For this review, take the finished solid that the model builds, in its own axes (mm). Coordinates: 2 decimals unless noted, no trailing zeros. Loops run counter-clockwise (first coordinate to the right, second up) from the corner with the lowest first, then second, coordinate; pieces in that order, holes last. Notation, with made-up numbers: (51, 44) - (74, 44) arc R21 cw to (74, 74) - close; hole circle Ø2 at (8.25, 75.5). An arc over 180 degrees is marked (long way). One line per item, written item: value. Start each with the question number.
1. To check wall thickness, follow line 1 (Z direction, x = 0, y = 5.25); line 2 (X direction, y = 2.95, z = 0); line 3 (X direction, y = 3, z = -10). State the ranges of each line that lie inside material, in increasing order. Write a range as from..to.
2. The part is to be moulded in two halves that separate along X. For faces 1 (the face through (6, 0, 0)), 2 (the face through (-29.97, 3.13, -1.32)), 3 (the face through (10.9, 4.2, -15.5)), say which applies: released by +X, released by -X, zero draft, split by the parting line, or undercut.
3. Take a section at B-B, the plane z = -10. State the section outline as (x, y) points, and give its area (3 significant figures).
4. Take a section at D-D, the plane y = 1. Count the separate pieces of the cut face and the enclosed holes in it, and give its area (3 significant figures).
5. Take a section at C-C, the plane x = 20. State the section outline as (y, z) points, and give its area (3 significant figures).
6. Take a section at A-A, the plane x = 0. State the section outline as (y, z) points, and give its area (3 significant figures).
7. Insertion check: pin 1 (2.5 mm diameter, centred on x = -20, z = 0, fed in from -Y); pin 2 (3 mm diameter, centred on y = 1.5, z = -23.5, fed in from +X); pin 3 (2 mm diameter, centred on y = 2, z = -9, fed in from -X); pin 4 (3 mm diameter, centred on x = 10.5, y = 5, fed in from -Z). Each pin has a flat end and moves straight along its axis. Give the tip position at first contact, or say it passes through.
```python
from build123d import *

# Parameters (mm, degrees)
SKETCH1_R             = 30
SKETCH1_R_2           = 1.89865
SKETCH1_R_3           = 1.9939
SKETCH1_R_4           = 4
BOSS_EXTRUDE1_DEPTH   = 6.35
CHAMFER1_SIZE         = 2.301024407
CHAMFER1_SIZE2        = 2.00025
CHAMFER1_PART_2_SIZE  = 2.301024407
CHAMFER1_PART_2_SIZE2 = 2.00025
CHAMFER1_PART_3_SIZE  = 2.301024407
CHAMFER1_PART_3_SIZE2 = 2.00025
CHAMFER1_PART_4_SIZE  = 2.301024407
CHAMFER1_PART_4_SIZE2 = 2.00025
CHAMFER1_PART_5_SIZE  = 2.301024407
CHAMFER1_PART_5_SIZE2 = 2.00025
CHAMFER1_PART_6_SIZE  = 2.301024407
CHAMFER1_PART_6_SIZE2 = 2.00025


with BuildPart() as part:
    # Sketch1 → Boss-Extrude1 (new body)
    with BuildSketch(Plane(origin=(0, 0, 0), x_dir=(1, 0, 0), z_dir=(0, 1, 0))):
        Circle(SKETCH1_R)
        with Locations((20, 0)):
            Circle(SKETCH1_R_2, mode=Mode.SUBTRACT)
        with Locations((10, -17.320508076)):
            Circle(SKETCH1_R_2, mode=Mode.SUBTRACT)
        with Locations((-10, -17.320508076)):
            Circle(SKETCH1_R_2, mode=Mode.SUBTRACT)
        with Locations((-20, 0)):
            Circle(SKETCH1_R_2, mode=Mode.SUBTRACT)
        with Locations((-10, 17.320508076)):
            Circle(SKETCH1_R_2, mode=Mode.SUBTRACT)
        with Locations((10, 17.320508076)):
            Circle(SKETCH1_R_2, mode=Mode.SUBTRACT)
        with Locations((0, 20)):
            Circle(SKETCH1_R_3, mode=Mode.SUBTRACT)
        with Locations((17.320508076, 10)):
            Circle(SKETCH1_R_3, mode=Mode.SUBTRACT)
        with Locations((17.320508076, -10)):
            Circle(SKETCH1_R_3, mode=Mode.SUBTRACT)
        with Locations((0, -20)):
            Circle(SKETCH1_R_3, mode=Mode.SUBTRACT)
        with Locations((-17.320508076, -10)):
            Circle(SKETCH1_R_3, mode=Mode.SUBTRACT)
        with Locations((-17.320508076, 10)):
            Circle(SKETCH1_R_3, mode=Mode.SUBTRACT)
        Circle(SKETCH1_R_4, mode=Mode.SUBTRACT)
    extrude(amount=BOSS_EXTRUDE1_DEPTH)

    # Chamfer1
    chamfer1_edges = [part.edges().sort_by_distance(p)[0] for p in [
        (8.10135, 6.35, 17.320508076),
    ]]
    chamfer1_side = [part.faces().sort_by_distance(p)[0] for p in [
        (8.10135, 3.175, 17.320508076),
    ]]
    chamfer(chamfer1_edges, length=CHAMFER1_SIZE, length2=CHAMFER1_SIZE2, reference=chamfer1_side[0])

    # Chamfer1 part 2
    chamfer1_part_2_edges = [part.edges().sort_by_distance(p)[0] for p in [
        (-11.89865, 6.35, 17.320508076),
    ]]
    chamfer1_part_2_side = [part.faces().sort_by_distance(p)[0] for p in [
        (-11.89865, 3.175, 17.320508076),
    ]]
    chamfer(chamfer1_part_2_edges, length=CHAMFER1_PART_2_SIZE, length2=CHAMFER1_PART_2_SIZE2, reference=chamfer1_part_2_side[0])

    # Chamfer1 part 3
    chamfer1_part_3_edges = [part.edges().sort_by_distance(p)[0] for p in [
        (-21.89865, 6.35, 0),
    ]]
    chamfer1_part_3_side = [part.faces().sort_by_distance(p)[0] for p in [
        (-21.89865, 3.175, 0),
    ]]
    chamfer(chamfer1_part_3_edges, length=CHAMFER1_PART_3_SIZE, length2=CHAMFER1_PART_3_SIZE2, reference=chamfer1_part_3_side[0])

    # Chamfer1 part 4
    chamfer1_part_4_edges = [part.edges().sort_by_distance(p)[0] for p in [
        (-11.89865, 6.35, -17.320508076),
    ]]
    chamfer1_part_4_side = [part.faces().sort_by_distance(p)[0] for p in [
        (-11.89865, 3.175, -17.320508076),
    ]]
    chamfer(chamfer1_part_4_edges, length=CHAMFER1_PART_4_SIZE, length2=CHAMFER1_PART_4_SIZE2, reference=chamfer1_part_4_side[0])

    # Chamfer1 part 5
    chamfer1_part_5_edges = [part.edges().sort_by_distance(p)[0] for p in [
        (8.10135, 6.35, -17.320508076),
    ]]
    chamfer1_part_5_side = [part.faces().sort_by_distance(p)[0] for p in [
        (8.10135, 3.175, -17.320508076),
    ]]
    chamfer(chamfer1_part_5_edges, length=CHAMFER1_PART_5_SIZE, length2=CHAMFER1_PART_5_SIZE2, reference=chamfer1_part_5_side[0])

    # Chamfer1 part 6
    chamfer1_part_6_edges = [part.edges().sort_by_distance(p)[0] for p in [
        (18.10135, 6.35, 0),
    ]]
    chamfer1_part_6_side = [part.faces().sort_by_distance(p)[0] for p in [
        (18.10135, 3.175, 0),
    ]]
    chamfer(chamfer1_part_6_edges, length=CHAMFER1_PART_6_SIZE, length2=CHAMFER1_PART_6_SIZE2, reference=chamfer1_part_6_side[0])


solid = part.part
```
Solutions:
1. line 1: -30..-21.99, -18.01..-4, 4..18.01, 21.99..30
1. line 2: -30..-21.9, -18.1..-4, 4..18.1, 21.9..30
1. line 3: -28.28..-19.31, -15.33..15.33, 19.31..28.28
2. face 1: zero draft
2. face 2: split by the parting line
2. face 3: undercut
3. outline: (-28.28, 0) - (-19.31, 0) - (-19.31, 6.35) - (-28.28, 6.35) - close; (-15.33, 0) - (15.33, 0) - (15.33, 6.35) - (-15.33, 6.35) - close; (19.31, 0) - (28.28, 0) - (28.28, 6.35) - (19.31, 6.35) - close
3. area: 309 mm2
4. separate pieces: 1
4. enclosed holes: 13
4. area: 2,630 mm2
5. outline: (0, -22.36) - (6.35, -22.36) - (6.35, -3.9) - (4.05, -1.9) - (0, -1.9) - close; (0, 1.9) - (4.05, 1.9) - (6.35, 3.9) - (6.35, 22.36) - (0, 22.36) - close
5. area: 255 mm2
6. outline: (0, -30) - (6.35, -30) - (6.35, -21.99) - (0, -21.99) - close; (0, -18.01) - (6.35, -18.01) - (6.35, -4) - (0, -4) - close; (0, 4) - (6.35, 4) - (6.35, 18.01) - (0, 18.01) - close; (0, 21.99) - (6.35, 21.99) - (6.35, 30) - (0, 30) - close
6. area: 280 mm2
7. pin 1: through
7. pin 2: x = 20.4
7. pin 3: x = -28.91
7. pin 4: z = -28.62
